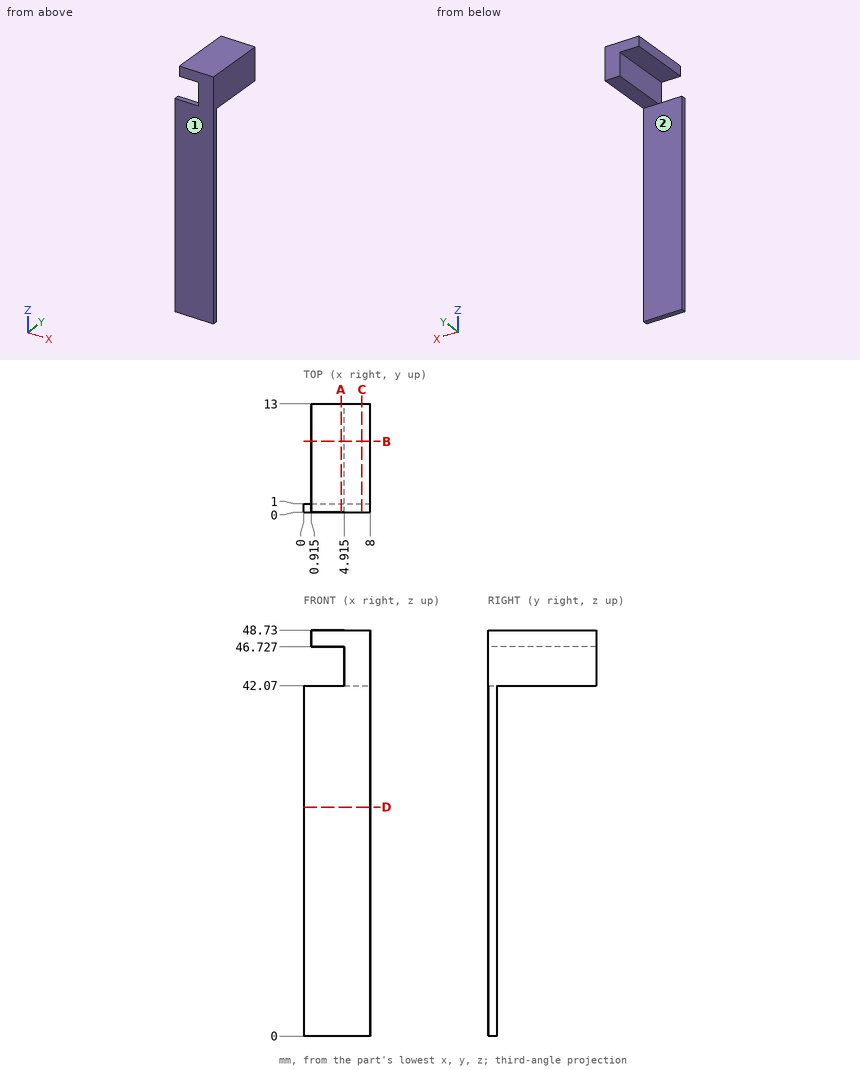
The figure shows three views and two pictorial views of one solid part (mm, origin at its lowest corner). Answer the questions. A direction names the side the tool comes from. Give positions to 0.01 mm unless a question says otherwise; leave off trailing zeros. Write each loop counter-clockwise with the first axis right and the second up, starting at its lowest first coordinate (ties: lowest second). Pieces come first, ordered by that corner, then holes. Notation, with made-up numbers: (-22.5, 66.5) - (-4.5, 66.5) arc R30 cw to (-4.5, 105.5) - close; hole circle Ø9 at (-25, -7). An arc over 180 degrees is marked (long way). Return JSON: item names as keys, results as strings.
Q1. A cutting plane is placed at B-B, the plane y = 8.5. Determine the outline of the cut face in (x, z) (1 decimal).
Reply:
{"outline": "(0.9, 46.7) - (4.9, 46.7) - (4.9, 42.1) - (8, 42.1) - (8, 48.7) - (0.9, 48.7) - close"}
Q2. A cutting plane is placed at C-C, the plane x = 7. Determine the outline of the cut face in (y, z).
Reply:
{"outline": "(0, 0) - (1, 0) - (1, 42.07) - (13, 42.07) - (13, 48.73) - (0, 48.73) - close"}
Q3. A cutting plane is placed at A-A, the plane x = 4.5. Determine the outline of the cut face in (y, z).
Reply:
{"outline": "(0, 0) - (1, 0) - (1, 42.07) - (0, 42.07) - close; (0, 46.73) - (13, 46.73) - (13, 48.73) - (0, 48.73) - close"}
Q4. A cutting plane is placed at D-D, the plane z = 27.5. Determine the outline of the cut face in (x, y).
Reply:
{"outline": "(0, 0) - (8, 0) - (8, 1) - (0, 1) - close"}
Q5. Given P1, Ø1.5, axis at y = 3, z = 11.5, coming from the -X side; P2, Ø1.5, axis at x = 4.5, z = 29.5, coming from the +Y side; P3, Ø1.5, axis at x = 7, y = 6, coming from the -Z side; P4, Ø2, axis at y = 9, z = 47.5, coming from the -X side (3 decimals), each flat-ended and moving along its own axis, determine where each tip first touches the part or whether it passes through.
Reply:
{"P1": "through", "P2": "y = 1", "P3": "z = 42.07", "P4": "x = 0.915"}
Q6. Consider line 1 along Z through (x, y) = (4.5, 0.75); line 2 along Y through (x, z) = (6.75, 35.5); line 3 along Z through (x, y) = (6.25, 2.5). Determine where each line is inside the solid, lowest interval first. Write a range as [from, to].
Reply:
{"line 1": "[0, 42.07], [46.73, 48.73]", "line 2": "[0, 1]", "line 3": "[42.07, 48.73]"}
Q7. For the marked faces 1 and 2, determine the directions among +Z, -Z, +X, -X, +Y, -Y from which every point of the face is accessible in a straight line to the end or side of a thin tool.
Reply:
{"face 1": "+Z, -Z, +X, -X, -Y", "face 2": "-Z, +X, -X, +Y"}
